Geometry check sheet. Reference: the model listing, model coordinates, mm. Give positions to 0.01 mm unless a question says otherwise; leave off trailing zeros. Write each loop counter-clockwise with the first axis right and the second up, starting at its lowest first coordinate (ties: lowest second). Pieces come first, ordered by that corner, then holes. Notation, with made-up numbers: (-8.5, 16) -> (32.5, 16) arc R14 ccw to (32.5, 37) -> close; hole circle Ø9 at (65, 86). An arc over 180 degrees is marked (long way). Write item = value, one per line. Start each with the question number.
1. Thickness scan on line 1 along X through (y, z) = (0, 0.2); line 2 along X through (y, z) = (0.5, 0.55); line 3 along Y through (x, z) = (11, 0.7). Record the ranges inside material, lowest first.
2. Cross-section at B-B, the plane z = 0.35. Record the cut outline in (x, y), plus the area to 3 significant figures.
3. Cross-section at C-C, the plane x = 11. Record the cut outline in (y, z).
4. Cross-section at A-A, the plane y = 2.25. Record the cut outline in (x, z).
5. Mould release check, pull along Y, two halves, no side actions. Record for faces 1 (the cylindrical face through (0.374, -9.996, 0.493)), 2 (the flat face through (17, 10.2, 0.5)), 3 (the cylindrical face through (12.464, 1.622, 0.493)): pulls with the +Y half, pulls with the -Y half, needs draft (parallel to the pull), parting line crosses it, or undercut.
6. Depth check by flat-ended pin: P1, Ø3, axis at x = -10.5, y = -4.5, coming from the -Z side. Enter the tip coordinate at first touch or a pass-through.
7. Cross-section at D-D, the plane y = 11. Record the cut outline in (x, z), plus the area to 3 significant figures.
Autodesk Inventor part; units mm, degrees
ref_plane "YZ Plane" through (0, 0, 0) normal (1, 0, 0) x (0, 1, 0)
ref_plane "XZ Plane" through (0, 0, 0) normal (0, 1, 0) x (-1, 0, 0)
ref_plane "XY Plane" through (0, 0, 0) normal (0, 0, 1) x (1, 0, 0)
sketch "Skizze1" plane through (0, 0, 0) normal (0, 0, 1) x (1, 0, 0)
  circle A0 centre (0, 25) radius 18.5 construction
  circle A1 centre (11, 1.2967) radius 1.5 construction
  circle A2 centre (-11, 1.2967) radius 1.5 construction
  circle A3 centre (0, 0) radius 5.5 construction
  arc A4 (-13.7171, 6) -> (-17.4753, 0.6301) centre (-13.7171, 2) ccw construction
  arc A5 (-17.4753, 0.6301) -> (17.4753, 0.6301) centre (0, 7) ccw construction
  arc A6 (17.4753, 0.6301) -> (13.7171, 6) centre (13.7171, 2) ccw construction
  line L0 (-13.7171, 6) -> (13.7171, 6) construction
  arc A7 (-15.4919, -4) -> (15.4919, -4) centre (0, 7) ccw construction
  arc A8 (-13.2288, 2.1205) -> (13.2288, 2.1205) centre (0, 7) ccw construction
  line L1 (-13.2288, 2.1205) -> (-13.2288, 18) construction
  line L2 (13.2288, 18) -> (-13.2288, 18) construction
  arc A9 (-19, 7) -> (-9.4721, -9.4705) centre (0, 7) ccw construction
  line L3 (-9.4721, -9.4705) -> (-9.4721, -18.6052) construction
  spline S0 degree 3 poles (-9.4721, -18.6052) (-10.8029, -18.1851) (-12.1032, -17.6649) (-16.3725, -15.5421) (-18.9977, -13.5189) (-21.2475, -11.0387) knots -1.506344 -1.506344 -1.506344 -1.506344 -1.083379 -1.083379 -0.074726 -0.074726 -0.074726 -0.074726 construction
  spline S1 degree 3 poles (-21.2475, -11.0387) (-21.4119, -10.8574) (-21.5695, -10.6702) (-21.8699, -10.2854) (-22.0126, -10.0879) (-22.148, -9.8855) knots -0.146464 -0.146464 -0.146464 -0.146464 -0.073068 -0.073068 0 0 0 0 construction
  spline S2 degree 3 poles (-22.148, -9.8855) (-24.4473, -6.4457) (-26.1085, -2.5959) (-28.9023, 6.7167) (-29.697, 12.4269) (-30, 18) knots -2.91726 -2.91726 -2.91726 -2.91726 -1.674385 -1.674385 0 0 0 0 construction
  line L4 (-30, 18) -> (-19, 18) construction
  line L5 (-19, 18) -> (-19, 7) construction
  line L6 (19, 18) -> (30, 18) construction
  spline S3 degree 3 poles (30, 18) (29.697, 12.4269) (28.9023, 6.7167) (26.1085, -2.5959) (24.4473, -6.4457) (22.148, -9.8855) knots -2.986913 -2.986913 -2.986913 -2.986913 -1.313902 -1.313902 -0.072047 -0.072047 -0.072047 -0.072047 construction
  spline S4 degree 3 poles (22.148, -9.8855) (22.0126, -10.0879) (21.8699, -10.2854) (21.5695, -10.6702) (21.4119, -10.8574) (21.2475, -11.0387) knots -0.146464 -0.146464 -0.146464 -0.146464 -0.073396 -0.073396 0 0 0 0 construction
  spline S5 degree 3 poles (21.2475, -11.0387) (19.6253, -12.8271) (17.7977, -14.3889) (13.7909, -16.9377) (11.6878, -17.9058) (9.4721, -18.6052) knots -3.300626 -3.300626 -3.300626 -3.300626 -3.030289 -3.030289 -2.770214 -2.770214 -2.770214 -2.770214 construction
  line L7 (9.4721, -18.6052) -> (9.4721, -9.4705) construction
  arc A10 (9.4721, -9.4705) -> (19, 7) centre (0, 7) ccw construction
  line L8 (19, 7) -> (19, 18) construction
  spline S6 degree 3 poles (21.2475, 47.0387) (21.4119, 46.8574) (21.5695, 46.6702) (21.8699, 46.2854) (22.0126, 46.0879) (22.148, 45.8855) knots -0.146464 -0.146464 -0.146464 -0.146464 -0.073068 -0.073068 0 0 0 0 construction
  spline S7 degree 3 poles (22.148, 45.8855) (24.4473, 42.4457) (26.1085, 38.5959) (28.9023, 29.2833) (29.697, 23.5731) (30, 18) knots -2.91726 -2.91726 -2.91726 -2.91726 -1.674385 -1.674385 0 0 0 0 construction
  line L9 (30, 18) -> (19, 18) construction
  line L10 (19, 18) -> (19, 29) construction
  arc A11 (19, 29) -> (9.4721, 45.4705) centre (0, 29) ccw construction
  line L11 (9.4721, 45.4705) -> (9.4721, 54.6052) construction
  spline S8 degree 3 poles (9.4721, 54.6052) (10.8029, 54.1851) (12.1032, 53.6649) (16.3725, 51.5421) (18.9977, 49.5189) (21.2475, 47.0387) knots -1.506344 -1.506344 -1.506344 -1.506344 -1.083379 -1.083379 -0.074726 -0.074726 -0.074726 -0.074726 construction
  spline S9 degree 3 poles (-22.148, 45.8855) (-22.0126, 46.0879) (-21.8699, 46.2854) (-21.5695, 46.6702) (-21.4119, 46.8574) (-21.2475, 47.0387) knots -0.146464 -0.146464 -0.146464 -0.146464 -0.073396 -0.073396 0 0 0 0 construction
  spline S10 degree 3 poles (-21.2475, 47.0387) (-19.6253, 48.8271) (-17.7977, 50.3889) (-13.7909, 52.9377) (-11.6878, 53.9058) (-9.4721, 54.6052) knots -3.300626 -3.300626 -3.300626 -3.300626 -3.030289 -3.030289 -2.770214 -2.770214 -2.770214 -2.770214 construction
  line L12 (-9.4721, 54.6052) -> (-9.4721, 45.4705) construction
  arc A12 (-9.4721, 45.4705) -> (-19, 29) centre (0, 29) ccw construction
  line L13 (-19, 29) -> (-19, 18) construction
  line L14 (-19, 18) -> (-30, 18) construction
  spline S11 degree 3 poles (-30, 18) (-29.697, 23.5731) (-28.9023, 29.2833) (-26.1085, 38.5959) (-24.4473, 42.4457) (-22.148, 45.8855) knots -2.986913 -2.986913 -2.986913 -2.986913 -1.313902 -1.313902 -0.072047 -0.072047 -0.072047 -0.072047 construction
  arc A13 (-17, 7) -> (17, 7) centre (0, 7) ccw
  arc A14 (-17, 13.5436) -> (17, 13.5436) centre (0, 25) ccw
  line L15 (17, 7) -> (17, 13.5436)
  line L16 (-17, 7) -> (-17, 13.5436)
  line L17 (0, 29) -> (0, 0) construction
  arc A15 (-13.8612, -2.8421) -> (13.8612, -2.8421) centre (0, 7) ccw construction
  circle A16 centre (0, 25) radius 20.5 construction
  line L18 (13.2288, 2.1205) -> (13.2288, 18)
  point P0 (0, 0)
  dimension "d2" = 2
  dimension "d3" = 2
extrude "Extrusion1" add sketch "Skizze1" along normal blind 1
sketch "Skizze2" plane through (0, 0, 1) normal (0, 0, 1) x (1, 0, 0)
  arc A0 (-17, 7) -> (17, 7) centre (0, 7) ccw
  line L0 (17, 7) -> (17, 13.5436)
  arc A1 (-17, 13.5436) -> (17, 13.5436) centre (0, 25) ccw
  line L1 (-17, 13.5436) -> (-17, 7)
  line L2 (17, 13.5436) -> (-17, 13.5436) construction
  line L3 (-17, 13.5436) -> (-17, -10) construction
  line L4 (-17, -10) -> (17, -10) construction
  line L5 (17, -10) -> (17, 13.5436) construction
  circle A2 centre (0, 25) radius 20.5 construction
  line L6 (-17, 13.5436) -> (17, 36.4564) construction
  line L7 (17, 13.5436) -> (17, 36.4564) construction
  point P0 (0, 0)
  point P1 (11, 1.2967)
  point P2 (0, 0)
  point P3 (-11, 1.2967)
  dimension "d6" = 6
  dimension "d7" = 17
  dimension "d8" = 28
  dimension "d9" = 12.2469
  dimension "d10" = 13.5436
  dimension "d11" = 23.5436
  dimension "d12" = 34
  dimension "d13" = 9.0436
  dimension "d14" = 6.5436
  dimension "d15" = 11.4564
  dimension "d16" = 20.5
  dimension "d17" = 17
  dimension "d18" = 22.9129
hole "Bohrung1" at (11, 1.2967, 1) at (-11, 1.2967, 1) direction (0, 0, -1) diameter 3 end through all
properties part number "minimalEncoder"
Answers:
q1.line_1 = -15.49 to -11.75, -10.25 to 10.25, 11.75 to 15.49
q1.line_2 = -15.71 to -12.27, -9.73 to 9.73, 12.27 to 15.71
q1.line_3 = -5.96 to -0.2, 2.8 to 7.7
q2.outline = (-17, 7) arc R17 ccw to (17, 7) -> (17, 13.54) arc R20.5 cw to (-17, 13.54) -> close; hole circle Ø3 at (-11, 1.3); hole circle Ø3 at (11, 1.3)
q2.area = 446 mm^2
q3.outline = (-5.96, 0) -> (-0.2, 0) -> (-0.2, 1) -> (-5.96, 1) -> close; (2.8, 0) -> (7.7, 0) -> (7.7, 1) -> (2.8, 1) -> close
q4.outline = (-16.32, 0) -> (-12.16, 0) -> (-12.16, 1) -> (-16.32, 1) -> close; (-9.84, 0) -> (9.84, 0) -> (9.84, 1) -> (-9.84, 1) -> close; (12.16, 0) -> (16.32, 0) -> (16.32, 1) -> (12.16, 1) -> close
q5.face_1 = pulls with the -Y half
q5.face_2 = needs draft
q5.face_3 = undercut
q6.P1 = 0
q7.outline = (-17, 0) -> (-14.97, 0) -> (-14.97, 1) -> (-17, 1) -> close; (14.97, 0) -> (17, 0) -> (17, 1) -> (14.97, 1) -> close
q7.area = 4.05 mm^2
